Work out the finished part from the listing and answer in its coordinate system (mm). A direction names the side the tool comes from. Coordinates: 2 decimals unless noted, no trailing zeros. Loops run counter-clockwise (first coordinate to the right, second up) from the corner with the lowest first, then second, coordinate; pieces in that order, holes last. Notation, with made-up numbers: (22.25, 59) -> (42.25, 59) arc R15 ccw to (42.25, 64) -> close; hole circle Ø6 at (81.25, 88). An arc over 180 degrees is marked (long way). Use a Markdown table: item, result. Add a question column.
```python
from build123d import *

# Parameters (mm, degrees)
SKETCH1_W           = 70
SKETCH1_H           = 20
SKETCH1_W_2         = 264.8
EXTRUDE_931_DEPTH   = 8
SKETCH2_W           = 36
SKETCH2_H           = 8
BOSS_EXTRUDE2_DEPTH = 8
SKETCH4_W           = 36
SKETCH4_H           = 8
BOSS_EXTRUDE3_DEPTH = 8
SKETCH5_R           = 1.5
CUT_EXTRUDE1_DEPTH  = 349.438631613
FILLET1_R           = 2.5
SKETCH6_W           = 30
SKETCH6_H           = 8
BOSS_EXTRUDE4_DEPTH = 30
SKETCH7_W           = 30
SKETCH7_H           = 8
BOSS_EXTRUDE5_DEPTH = 30
SKETCH8_W           = 8
SKETCH8_H           = 50
CUT_EXTRUDE2_DEPTH  = 356.142619239
SKETCH11_R          = 1.65
CUT_EXTRUDE3_DEPTH  = 356.142619239


with BuildPart() as part:
    # Sketch1 → Extrude 931 (new body)
    with BuildSketch(Plane(origin=(0, 0, 0), x_dir=(1, 0, 0), z_dir=(0, 1, 0))):
        with Locations((-35, -78.2)):
            Rectangle(SKETCH1_W, SKETCH1_H)
        with Locations((132.4, -78.2)):
            Rectangle(SKETCH1_W_2, SKETCH1_H)
        with Locations((299.8, -78.2)):
            Rectangle(SKETCH1_W, SKETCH1_H)
    extrude(amount=EXTRUDE_931_DEPTH)

    # Sketch2 → Boss-Extrude2 (add)
    with BuildSketch(Plane(origin=(0, 0, 68.2), x_dir=(-1, 0, 0), z_dir=(0, 0, -1))):
        with Locations((0, 4)):
            Rectangle(SKETCH2_W, SKETCH2_H)
        with Locations((-300, 4)):
            Rectangle(SKETCH2_W, SKETCH2_H)
    extrude(amount=BOSS_EXTRUDE2_DEPTH)

    # Sketch4 → Boss-Extrude3 (add)
    with BuildSketch(Plane.XY.offset(88.2)):
        with Locations((0, 4)):
            Rectangle(SKETCH4_W, SKETCH4_H)
        with Locations((300, 4)):
            Rectangle(SKETCH4_W, SKETCH4_H)
    extrude(amount=BOSS_EXTRUDE3_DEPTH)

    # Sketch5 → Cut-Extrude1 (cut, through all)
    with BuildSketch(Plane(origin=(0, 8, 0), x_dir=(1, 0, 0), z_dir=(0, 1, 0))):
        with Locations(Location((-13.4, -91.6, 0), (0, 0, 270))):
            Circle(SKETCH5_R)
        with Locations(Location((13.4, -91.6, 0), (0, 0, 270))):
            Circle(SKETCH5_R)
        with Locations(Location((13.4, -64.8, 0), (0, 0, 270))):
            Circle(SKETCH5_R)
        with Locations(Location((-13.4, -64.8, 0), (0, 0, 270))):
            Circle(SKETCH5_R)
        with Locations(Location((313.4, -91.6, 0), (0, 0, 270))):
            Circle(SKETCH5_R)
        with Locations(Location((286.6, -64.8, 0), (0, 0, 270))):
            Circle(SKETCH5_R)
        with Locations(Location((313.4, -64.8, 0), (0, 0, 270))):
            Circle(SKETCH5_R)
        with Locations(Location((286.6, -91.6, 0), (0, 0, 270))):
            Circle(SKETCH5_R)
    extrude(amount=-CUT_EXTRUDE1_DEPTH, mode=Mode.SUBTRACT)

    # Fillet1
    fillet1_edges = [part.edges().sort_by_distance(p)[0] for p in [
        (-18, 4, 60.2),
        (18, 4, 60.2),
        (318, 4, 60.2),
        (18, 4, 96.2),
        (-18, 4, 96.2),
        (318, 4, 96.2),
    ]]
    fillet(fillet1_edges, radius=FILLET1_R)

    # Sketch6 → Boss-Extrude4 (add)
    with BuildSketch(Plane.XY.offset(88.2)):
        with Locations((267, 4)):
            Rectangle(SKETCH6_W, SKETCH6_H)
    extrude(amount=BOSS_EXTRUDE4_DEPTH)

    # Sketch7 → Boss-Extrude5 (add)
    with BuildSketch(Plane(origin=(0, 0, 68.2), x_dir=(-1, 0, 0), z_dir=(0, 0, -1))):
        with Locations((-267, 4)):
            Rectangle(SKETCH7_W, SKETCH7_H)
    extrude(amount=BOSS_EXTRUDE5_DEPTH)

    # Sketch8 → Cut-Extrude2 (cut, through all)
    with BuildSketch(Plane(origin=(0, 8, 0), x_dir=(1, 0, 0), z_dir=(0, 1, 0))):
        with Locations((267, -78.2)):
            Rectangle(SKETCH8_W, SKETCH8_H)
    extrude(amount=-CUT_EXTRUDE2_DEPTH, mode=Mode.SUBTRACT)

    # Sketch11 → Cut-Extrude3 (cut, through all)
    with BuildSketch(Plane(origin=(0, 8, 0), x_dir=(1, 0, 0), z_dir=(0, 1, 0))):
        with Locations(Location((258, -114.2, 0), (0, 0, 270))):
            Circle(SKETCH11_R)
        with Locations(Location((258, -82.2, 0), (0, 0, 270))):
            Circle(SKETCH11_R)
    extrude(amount=-CUT_EXTRUDE3_DEPTH, mode=Mode.SUBTRACT)


solid = part.part
```
Item 1: Section B-B (x = 68) is taken. Determine the outline of the cut face in (y, z).
Item 2: Given pin 1 (5 mm diameter, centred on x = 313.4, z = 91.6, fed in from -Y); pin 2 (1 mm diameter, centred on x = 100.5, y = 1, fed in from -Z); pin 3 (4 mm diameter, centred on x = 329.5, y = 3, fed in from +Z); pin 4 (2.5 mm diameter, centred on x = 313.4, z = 64.8, fed in from +Y), each flat-ended and moving along its own axis, determine where each tip first touches the part or whether it passes through.
Item 3: For faces 4 (the face through (-44, 4, 88.2)), 5 (the face through (263, 4, 79)), 6 (the face through (299, 4, 96.2)), 7 (the face through (252, 4, 53)), determine the directions among +Z, -Z, +X, -X, +Y, -Y from which every point of the face is accessible in a straight line to the end or side of a thin tool.
Item 4: For a pull along X with two mould halves and no side action, classify faces 1 (the face through (282, 4, 49)), 2 (the face through (327, 4, 68.2)), 3 (the face through (271, 4, 79)) as +X half, -X half, draft (parallel to the pull), parting line (faces both ways), or undercut.
Item 5: Section A-A (y = 2) is taken. Count the separate pieces of the cut face and the enclosed holes in it, then the cut area to 3 significant figures.
Item 6: Find the intervals of material crossed by probe 1 along Z at (x, y) = (313.4, 4); probe 2 along Z at (x, y) = (258, 2.5); probe 3 along X at (y, z) = (2.75, 82.2), in increasing order.
Output:
| question | item | result |
|---|---|---|
| 1 | outline | (0, 68.2) -> (8, 68.2) -> (8, 88.2) -> (0, 88.2) -> close |
| 2 | pin 1 | stops at y = 0 |
| 2 | pin 2 | stops at z = 68.2 |
| 2 | pin 3 | stops at z = 88.2 |
| 2 | pin 4 | passes through |
| 3 | face 4 | +Z, -X, +Y, -Y |
| 3 | face 5 | +Y, -Y |
| 3 | face 6 | +Z, +X, +Y, -Y |
| 3 | face 7 | -Z, +Y, -Y |
| 4 | face 1 | +X half |
| 4 | face 2 | draft |
| 4 | face 3 | undercut |
| 5 | separate pieces | 1 |
| 5 | enclosed holes | 11 |
| 5 | area | 10,600 mm2 |
| 6 | probe 1 | z = 60.2 to 63.3, 66.3 to 90.1, 93.1 to 96.2 |
| 6 | probe 2 | z = 38.2 to 80.55, 83.85 to 112.55, 115.85 to 118.2 |
| 6 | probe 3 | x = -70 to 256.35, 259.65 to 263, 271 to 334.8 |
